Read the model definition and answer for the solid it produces. Units are mm, in the model's axes. A direction names the side the tool comes from. Coordinates: 2 decimals unless noted, no trailing zeros. Write each loop counter-clockwise with the first axis right and the second up, starting at its lowest first coordinate (ties: lowest second). Pieces come first, ordered by that corner, then holes. Notation, with made-up numbers: (16, 58) -> (66, 58) arc R25 cw to (66, 94) -> close; hole circle Ø11 at (3, 66). An arc over 180 degrees is marked (long way). Answer in a Markdown table with one row per item. Add a question column.
Item 1: Straight lines are drawn through the part: line 1 (Y direction, x = 0.45, z = -1.15); line 2 (Y direction, x = -2.45, z = 1.25); line 3 (Z direction, x = -0.05, y = -2.75). For each, find the intervals that lie inside material, in ascending order. Write a range as from..to.
Item 2: Given pin 1 Ø1 at (y, z) = (0.5, -0.5) entering from -X; pin 2 Ø1.5 at (y, z) = (0.5, -2) entering from -X; pin 3 Ø1 at (x, y) = (0.5, -5) entering from +Z, each flat-ended and moving along its own axis, determine where each tip first touches the part or whether it passes through.
Item 3: Section A-A on x = 0 is taken. Write down the section's boundary in (y, z), then the cut area to 3 significant figures.
Item 4: Which of the six approach directions +Z, -Z, +X, -X, +Y, -Y give full straight-line access (tool end or side, diameter ignored) to faces 4 (the face through (1.08, 1.86, 0.63)), 5 (the face through (0, -6, 0)), 6 (the face through (-1.5, -2.96, 0.07))?
Item 5: Section B-B on y = -0.75 is taken. Write down the section's boundary in (x, z), then the cut area to 3 significant figures.
Item 6: For a pull along X with two mould halves and no side action, classify faces 1 (the face through (-3, 2, 0)), 2 (the face through (0, 1.2, 0)), 3 (the face through (1.3, 2.5, 0.6)) as +X half, -X half, draft (parallel to the pull), parting line (faces both ways), or undercut.
```python
from build123d import *

# Parameters (mm, degrees)
SKETCH_1_R            = 3
EXTRUDE_251_DEPTH     = 2.5
CHAMFER_1_SIZE        = 1.5
CUT_EXTRUDE_459_DEPTH = 1.3
SKETCH_3_R            = 1.5
EXTRUDE_571_DEPTH     = 6


with BuildPart() as part:
    # 草图1 → Extrude 251 (new body)
    with BuildSketch(Plane(origin=(0, 0, 0), x_dir=(1, 0, 0), z_dir=(0, 1, 0))):
        Circle(SKETCH_1_R)
    extrude(amount=EXTRUDE_251_DEPTH)

    # 倒角1
    chamfer_1_edges = [part.edges().sort_by_distance(p)[0] for p in [
        (-3, 0, 0),
    ]]
    chamfer(chamfer_1_edges, length=CHAMFER_1_SIZE)

    # 草图2 → Cut-Extrude 459 (cut)
    with BuildSketch(Plane(origin=(0, 2.5, 0), x_dir=(1, 0, 0), z_dir=(0, 1, 0))):
        Polygon((1.443375673, 0), (0.721687836, 1.25), (-0.721687836, 1.25), (-1.443375673, 0), (-0.721687836, -1.25), (0.721687836, -1.25), align=None)
    extrude(amount=-CUT_EXTRUDE_459_DEPTH, mode=Mode.SUBTRACT)

    # 草图3 → Extrude 571 (add)
    with BuildSketch(Plane.XZ):
        Circle(SKETCH_3_R)
    extrude(amount=EXTRUDE_571_DEPTH)


solid = part.part
```
Results below:
| question | item | result |
|---|---|---|
| 1 | line 1 | y = -6..1.2 |
| 1 | line 2 | y = 1.25..2.5 |
| 1 | line 3 | z = -1.5..1.5 |
| 2 | pin 1 | stops at x = -2.46 |
| 2 | pin 2 | stops at x = -2.09 |
| 2 | pin 3 | stops at z = 1.5 |
| 3 | outline | (-6, -1.5) -> (0, -1.5) -> (1.5, -3) -> (2.5, -3) -> (2.5, -1.25) -> (1.2, -1.25) -> (1.2, 1.25) -> (2.5, 1.25) -> (2.5, 3) -> (1.5, 3) -> (0, 1.5) -> (-6, 1.5) -> close |
| 3 | area | 27.5 mm2 |
| 4 | face 4 | +Y |
| 4 | face 5 | +Z, -Z, +X, -X, -Y |
| 4 | face 6 | -Y |
| 5 | outline | circle Ø3 at (0, 0) |
| 5 | area | 7.07 mm2 |
| 6 | face 1 | parting line |
| 6 | face 2 | undercut |
| 6 | face 3 | draft |
